from build123d import *

# Parameters (mm, degrees)
BOSS_EXTRUDE1_START = -73.5
SKETCH1_W           = 11
SKETCH1_H           = 6
BOSS_EXTRUDE1_DEPTH = 124
SKETCH2_W           = 11
SKETCH2_H           = 6
BOSS_EXTRUDE3_DEPTH = 15
FILLET1_R           = 7.5
SKETCH4_R           = 5.5
BOSS_EXTRUDE4_DEPTH = 5
SKETCH5_R           = 6.75
BOSS_EXTRUDE5_DEPTH = 1.5
FILLET2_R           = 0.5
SKETCH6_R           = 1.75
CUT_EXTRUDE1_DEPTH  = 3
FILLET3_R           = 0.25


with BuildPart() as part:
    # Sketch1 → Boss-Extrude1 (new body)
    with BuildSketch(Plane(origin=(0, 0, 0), x_dir=(0, 0, -1), z_dir=(1, 0, 0)).offset(BOSS_EXTRUDE1_START)):
        with Locations((5.5, -3)):
            Rectangle(SKETCH1_W, SKETCH1_H)
    extrude(amount=BOSS_EXTRUDE1_DEPTH)

    # Sketch2 → Boss-Extrude3 (add)
    # profile 1 of 2: a face of its own
    with BuildSketch(Plane(origin=(50.5, 0, 0), x_dir=(0, 0, -1), z_dir=(1, 0, 0))):
        Polygon((-5, 8.5), (-5, -9), (40, -9), (40, 28.5), (23, 28.5), (23, 23.5), (9, 23.5), (9, 8.5), align=None)
        with Locations((5.5, -3)):
            Rectangle(SKETCH2_W, SKETCH2_H, mode=Mode.SUBTRACT)
    # profile 2 of 2: a face of its own
    with BuildSketch(Plane(origin=(50.5, 0, 0), x_dir=(0, 0, -1), z_dir=(1, 0, 0))):
        with Locations((5.5, -3)):
            Rectangle(SKETCH2_W, SKETCH2_H)
    extrude(amount=BOSS_EXTRUDE3_DEPTH)

    # Fillet1
    # the kernel refuses this fillet: 7.5 mm, written as the material it takes off along each edge
    with BuildSketch(Plane(origin=(50.5, 27.25, 5), x_dir=(1, 0, 0), z_dir=(0, -1, 0))) as fillet1_piece_1_section:
        with BuildLine():
            CenterArc((FILLET1_R, -FILLET1_R), FILLET1_R, 90, 90)
            Line((0, -FILLET1_R), (0, 0))
            Line((0, 0), (FILLET1_R, 0))
        make_face()
    fillet1_piece_1 = extrude(amount=55, mode=Mode.PRIVATE)
    fillet1_piece_1 = split(fillet1_piece_1, bisect_by=Plane(origin=(52.221902298, 4.25, 0), z_dir=(0, 0, 1)), keep=Keep.TOP, mode=Mode.PRIVATE)
    add(fillet1_piece_1, mode=Mode.SUBTRACT)
    with BuildSketch(Plane(origin=(50.5, 27.25, 5), x_dir=(1, 0, 0), z_dir=(0, -1, 0))) as fillet1_piece_2_section:
        with BuildLine():
            CenterArc((FILLET1_R, -FILLET1_R), FILLET1_R, 90, 90)
            Line((0, -FILLET1_R), (0, 0))
            Line((0, 0), (FILLET1_R, 0))
        make_face()
    fillet1_piece_2 = extrude(amount=55, mode=Mode.PRIVATE)
    fillet1_piece_2 = split(fillet1_piece_2, bisect_by=Plane(origin=(50.628023306, 0, -0.621369721), z_dir=(0, 1, 0)), keep=Keep.TOP, mode=Mode.PRIVATE)
    add(fillet1_piece_2, mode=Mode.SUBTRACT)
    with BuildSketch(Plane(origin=(50.5, 27.25, 5), x_dir=(1, 0, 0), z_dir=(0, -1, 0))) as fillet1_piece_3_section:
        with BuildLine():
            CenterArc((FILLET1_R, -FILLET1_R), FILLET1_R, 90, 90)
            Line((0, -FILLET1_R), (0, 0))
            Line((0, 0), (FILLET1_R, 0))
        make_face()
    fillet1_piece_3 = extrude(amount=55, mode=Mode.PRIVATE)
    fillet1_piece_3 = split(fillet1_piece_3, bisect_by=Plane(origin=(50.628023306, -6, -0.621369721), z_dir=(0, -1, 0)), keep=Keep.TOP, mode=Mode.PRIVATE)
    add(fillet1_piece_3, mode=Mode.SUBTRACT)
    with BuildSketch(Plane(origin=(65.5, 27.25, 5), x_dir=(-1, 0, 0), z_dir=(0, -1, 0))) as fillet1_piece_4:
        with BuildLine():
            CenterArc((FILLET1_R, FILLET1_R), FILLET1_R, 180, 90)
            Line((0, FILLET1_R), (0, 0))
            Line((0, 0), (FILLET1_R, 0))
        make_face()
    extrude(amount=55, mode=Mode.SUBTRACT)
    with BuildSketch(Plane(origin=(50.5, 42.25, -9), x_dir=(0, 0, -1), z_dir=(0, -1, 0))) as fillet1_piece_5:
        with BuildLine():
            CenterArc((FILLET1_R, FILLET1_R), FILLET1_R, 180, 90)
            Line((0, FILLET1_R), (0, 0))
            Line((0, 0), (FILLET1_R, 0))
        make_face()
    extrude(amount=33.75, mode=Mode.SUBTRACT)
    with BuildSketch(Plane(origin=(65.5, 42.25, -9), x_dir=(0, 0, -1), z_dir=(0, -1, 0))) as fillet1_piece_6:
        with BuildLine():
            CenterArc((FILLET1_R, -FILLET1_R), FILLET1_R, 90, 90)
            Line((0, -FILLET1_R), (0, 0))
            Line((0, 0), (FILLET1_R, 0))
        make_face()
    extrude(amount=33.75, mode=Mode.SUBTRACT)
    with BuildSketch(Plane(origin=(50.5, -27.75, -40), x_dir=(0, 0, 1), z_dir=(0, 1, 0))) as fillet1_piece_7:
        with BuildLine():
            CenterArc((FILLET1_R, FILLET1_R), FILLET1_R, 180, 90)
            Line((0, FILLET1_R), (0, 0))
            Line((0, 0), (FILLET1_R, 0))
        make_face()
    extrude(amount=75, mode=Mode.SUBTRACT)
    with BuildSketch(Plane(origin=(65.5, -27.75, -40), x_dir=(0, 0, 1), z_dir=(0, 1, 0))) as fillet1_piece_8:
        with BuildLine():
            CenterArc((FILLET1_R, -FILLET1_R), FILLET1_R, 90, 90)
            Line((0, -FILLET1_R), (0, 0))
            Line((0, 0), (FILLET1_R, 0))
        make_face()
    extrude(amount=75, mode=Mode.SUBTRACT)

    # Sketch4 → Boss-Extrude4 (add)
    with BuildSketch(Plane(origin=(0, 23.5, 0), x_dir=(1, 0, 0), z_dir=(0, 1, 0))):
        with Locations(Location((58, 16, 0), (0, 0, 270))):
            Circle(SKETCH4_R)
    extrude(amount=BOSS_EXTRUDE4_DEPTH)

    # Sketch5 → Boss-Extrude5 (add)
    with BuildSketch(Plane(origin=(0, 28.5, 0), x_dir=(1, 0, 0), z_dir=(0, 1, 0))):
        with Locations(Location((58, 16, 0), (0, 0, 270))):
            Circle(SKETCH5_R)
    extrude(amount=-BOSS_EXTRUDE5_DEPTH)

    # Fillet2
    fillet2_edges = [part.edges().sort_by_distance(p)[0] for p in [
        (58, 27, -22.75),
        (58, 28.5, -22.75),
    ]]
    fillet(fillet2_edges, radius=FILLET2_R)

    # Sketch6 → Cut-Extrude1 (cut)
    with BuildSketch(Plane(origin=(0, 8.5, 0), x_dir=(1, 0, 0), z_dir=(0, 1, 0))):
        with Locations(Location((58, 2.5, 0), (0, 0, 270))):
            Circle(SKETCH6_R)
    extrude(amount=-CUT_EXTRUDE1_DEPTH, mode=Mode.SUBTRACT)

    # Fillet3
    fillet3_edges = [part.edges().sort_by_distance(p)[0] for p in [
        (58, 5.5, -4.25),
        (58, 8.5, -4.25),
    ]]
    fillet(fillet3_edges, radius=FILLET3_R)


solid = part.part
Source: CAD feature listing. Evaluate the final solid. Frame: model axes, mm. A direction names the side the tool comes from. Give positions to 0.01 mm unless a question says otherwise; leave off trailing zeros. Order: outer loops, then holes, each group sorted by start corner. A loop starts at its lowest first (then second) coordinate and runs counter-clockwise, first axis right, second up. Notation, with made-up numbers: (-16.75, -23.75) -> (10.25, -23.75) arc R23 cw to (10.25, -2.75) -> close; hole circle Ø3 at (16.5, 14). An arc over 180 degrees is marked (long way). Write item = value, one per line.
Q1. Cut plane B-B, the plane y = -2.5. Output: boundary loops of the cut face in (x, z), and give its area (3 significant figures).
Data:
outline = (-73.5, -11) -> (50.5, -11) -> (50.5, -32.5) arc R7.5 ccw to (65.5, -32.5) -> (65.5, -2.5) arc R7.5 ccw to (50.93, 0) -> (-73.5, 0) -> close
area = 1,990 mm^2
Q2. Pull-direction query (Z, two-part tool) for faces 1 (the face through (61, 23.5, -21)), 2 (the face through (-73.5, -3, -5)), 3 (the face through (-12, -3, -11)), 4 (the face through (58, 16, -9)); classes: released by +Z, released by -Z, zero draft, split by the parting line, or undercut.
Data:
face_1 = undercut
face_2 = zero draft
face_3 = released by -Z
face_4 = released by +Z
Q3. Cut plane D-D, the plane y = 22. Output: boundary loops of the cut face in (x, z).
Data:
outline = (50.5, -32.5) arc R7.5 ccw to (65.5, -32.5) -> (65.5, -16.5) arc R7.5 ccw to (50.5, -16.5) -> close
Q4. Material intervals for line 1 (X direction, y = 7.75, z = -2.5); line 2 (X direction, y = 7, z = -6.5); line 3 (Y direction, x = 47, z = -3), sorted ascending. Write a range as from..to.
Data:
line_1 = 50.5..56.25, 59.75..65.5
line_2 = 50.5..65.5
line_3 = -6..0
Q5. Cut plane C-C, the plane z = -25.5. Output: boundary loops of the cut face in (x, y).
Data:
outline = (50.5, -9) -> (65.5, -9) -> (65.5, 28.5) -> (50.5, 28.5) -> close
Q6. Cut plane A-A, the plane x = 58. Output: boundary loops of the cut face in (y, z), and give its area (3 significant figures).
Data:
outline = (-9, -40) -> (28.5, -40) -> (28.5, -23) -> (23.5, -23) -> (23.5, -21.5) -> (27, -21.5) -> (27, -22.25) arc R0.5 ccw to (27.5, -22.75) -> (28, -22.75) arc R0.5 ccw to (28.5, -22.25) -> (28.5, -9.75) arc R0.5 ccw to (28, -9.25) -> (27.5, -9.25) arc R0.5 ccw to (27, -9.75) -> (27, -10.5) -> (23.5, -10.5) -> (23.5, -9) -> (8.5, -9) -> (8.5, -4.5) arc R0.25 ccw to (8.25, -4.25) -> (5.75, -4.25) arc R0.25 cw to (5.5, -4) -> (5.5, -1) arc R0.25 cw to (5.75, -0.75) -> (8.25, -0.75) arc R0.25 ccw to (8.5, -0.5) -> (8.5, 5) -> (-9, 5) -> close
area = 1,390 mm^2
Q7. Set-up query: faces 5 (the face through (-12, -6, -5)), 6 (the face through (58, 26, -23)), 7 (the face through (-10, 0, -6)), 8 (the face through (58, 5.5, -3)). Return all of +Z, -Z, +X, -X, +Y, -Y with unobstructed straight access to the full face (end or side cutting, diameter ignored); none if empty.
Data:
face_5 = +Z, -Z, -X, -Y
face_6 = +X, -X, +Y
face_7 = +Z, -Z, -X, +Y
face_8 = +Y
Q8. Pin query (flat end, axial travel): pin 1 (5.5 mm diameter, centred on x = -34, z = -5, fed in from +Y); pin 2 (2.5 mm diameter, centred on x = 57, y = 25.5, fed in from +Z); pin 3 (6.5 mm diameter, centred on x = -19.5, y = -3.5, fed in from +Z). Return the tip coordinate at first contact, or that it passes through.
Data:
pin_1 = 0
pin_2 = -10.5
pin_3 = 0
